from build123d import *

# Parameters (mm, degrees)
BOSS_EXTRUDE1_DEPTH      = 88.9
BOSS_EXTRUDE1_DEPTH_BACK = 88.9
SKETCH2_R                = 3.3782
CUT_EXTRUDE2_DEPTH       = 163.899847125
SKETCH5_R                = 14.2875
SKETCH5_R_2              = 3.3782
CUT_EXTRUDE3_DEPTH       = 164.564592404
BOSS_EXTRUDE3_START      = -19.05
BOSS_EXTRUDE3_DEPTH      = 201.6125
CONVERT_SOLID1_START     = -88.9
CONVERT_SOLID1_DEPTH     = 177.8
CONVERT_SOLID1_START_2   = -103.98125
CONVERT_SOLID1_2_DEPTH   = 201.6125
CONVERT_SOLID1_3_DEPTH   = 177.8
CONVERT_SOLID1_4_DEPTH   = 201.6125
SKETCH7_R                = 3.3782
CUT_EXTRUDE4_DEPTH       = 185.298076003


# Read off the part's stored shape, not the designer's step: Convert-Solid1
with BuildPart() as part:
    # Sketch1 → Boss-Extrude1 (new, two sides: drawn at the far end of the back side and taken through both)
    with BuildSketch(Plane(origin=(0, 0, 0), x_dir=(0, 0, -1), z_dir=(1, 0, 0)).offset(-BOSS_EXTRUDE1_DEPTH_BACK)):
        Polygon((-132.55625, -29.4132), (-132.55625, -32.5882), (-113.50625, -32.5882), (-113.50625, 0), (113.50625, 0), (113.50625, -32.5882), (132.55625, -32.5882), (132.55625, -29.4132), (116.68125, -29.4132), (116.68125, 3.175), (-116.68125, 3.175), (-116.68125, -29.4132), align=None)
    extrude(amount=BOSS_EXTRUDE1_DEPTH + BOSS_EXTRUDE1_DEPTH_BACK)

    # Sketch2 → Cut-Extrude2 (cut, through all)
    with BuildSketch(Plane(origin=(0, -29.4132, 0), x_dir=(1, 0, 0), z_dir=(0, 1, 0))):
        with Locations(Location((-76.2, -124.61875, 0), (0, 0, 270))):
            Circle(SKETCH2_R)
        with Locations(Location((0, -124.61875, 0), (0, 0, 270))):
            Circle(SKETCH2_R)
        with Locations(Location((76.2, -124.61875, 0), (0, 0, 270))):
            Circle(SKETCH2_R)
        with Locations(Location((76.2, 124.61875, 0), (0, 0, 90))):
            Circle(SKETCH2_R)
        with Locations(Location((0, 124.61875, 0), (0, 0, 90))):
            Circle(SKETCH2_R)
        with Locations(Location((-76.2, 124.61875, 0), (0, 0, 90))):
            Circle(SKETCH2_R)
    extrude(amount=-CUT_EXTRUDE2_DEPTH, mode=Mode.SUBTRACT)

    # Sketch5 → Cut-Extrude3 (cut, through all)
    with BuildSketch(Plane(origin=(0, 3.175, 0), x_dir=(1, 0, 0), z_dir=(0, 1, 0))):
        with Locations(Location((0, 12.7, 0), (0, 0, 270))):
            Circle(SKETCH5_R)
        with Locations(Location((-70.612, 83.312, 0), (0, 0, 270))):
            Circle(SKETCH5_R_2)
        with Locations(Location((70.612, 83.312, 0), (0, 0, 270))):
            Circle(SKETCH5_R_2)
        with Locations(Location((70.612, -57.912, 0), (0, 0, 270))):
            Circle(SKETCH5_R_2)
        with Locations(Location((-70.612, -57.912, 0), (0, 0, 270))):
            Circle(SKETCH5_R_2)
    extrude(amount=-CUT_EXTRUDE3_DEPTH, mode=Mode.SUBTRACT)

    # Sketch6 → Boss-Extrude3 (add)
    with BuildSketch(Plane.XY.offset(116.68125).offset(BOSS_EXTRUDE3_START)):
        Polygon((88.9, 3.175), (107.95, 3.175), (107.95, -29.4132), (123.825, -29.4132), (123.825, -32.5882), (104.775, -32.5882), (104.775, 0), (88.9, 0), align=None)
        Polygon((-88.9, 0), (-88.9, 3.175), (-107.95, 3.175), (-107.95, -29.4132), (-123.825, -29.4132), (-123.825, -32.5882), (-104.775, -32.5882), (-104.775, 0), align=None)
    extrude(amount=-BOSS_EXTRUDE3_DEPTH)

    # Convert-Solid1 outline → Convert-Solid1 (add)
    with BuildSketch(Plane.YZ.offset(CONVERT_SOLID1_START)):
        with BuildLine():
            Line((-29.4132, -116.68125), (-29.4132, -117.95125))
            ThreePointArc((-29.4132, -117.95125), (-29.041225612, -117.053224388), (-28.1432, -116.68125))
            Line((-28.1432, -116.68125), (-29.4132, -116.68125))
        make_face()
        with BuildLine():
            Line((0, -113.50625), (0, -112.23625))
            ThreePointArc((0, -112.23625), (-0.371974388, -113.134275612), (-1.27, -113.50625))
            Line((-1.27, -113.50625), (0, -113.50625))
        make_face()
        with BuildLine():
            ThreePointArc((-1.27, 113.50625), (-0.371974388, 113.134275612), (0, 112.23625))
            Line((0, 112.23625), (0, 113.50625))
            Line((0, 113.50625), (-1.27, 113.50625))
        make_face()
        with BuildLine():
            Line((-29.4132, 116.68125), (-28.1432, 116.68125))
            ThreePointArc((-28.1432, 116.68125), (-29.041225612, 117.053224388), (-29.4132, 117.95125))
            Line((-29.4132, 117.95125), (-29.4132, 116.68125))
        make_face()
    extrude(amount=CONVERT_SOLID1_DEPTH)

    # Convert-Solid1 2 outline → Convert-Solid1 2 (add)
    with BuildSketch(Plane.XY.offset(CONVERT_SOLID1_START_2)):
        with BuildLine():
            Line((107.95, -29.4132), (109.22, -29.4132))
            ThreePointArc((109.22, -29.4132), (108.321974388, -29.041225612), (107.95, -28.1432))
            Line((107.95, -28.1432), (107.95, -29.4132))
        make_face()
        with BuildLine():
            Line((-107.95, -29.4132), (-107.95, -28.1432))
            ThreePointArc((-107.95, -28.1432), (-108.321974388, -29.041225612), (-109.22, -29.4132))
            Line((-109.22, -29.4132), (-107.95, -29.4132))
        make_face()
        with BuildLine():
            ThreePointArc((-104.775, -1.27), (-104.403025612, -0.371974388), (-103.505, 0))
            Line((-103.505, 0), (-104.775, 0))
            Line((-104.775, 0), (-104.775, -1.27))
        make_face()
        with BuildLine():
            ThreePointArc((103.505, 0), (104.403025612, -0.371974388), (104.775, -1.27))
            Line((104.775, -1.27), (104.775, 0))
            Line((104.775, 0), (103.505, 0))
        make_face()
    extrude(amount=CONVERT_SOLID1_2_DEPTH)

    # Convert-Solid1 3 outline → Convert-Solid1 3 (cut)
    with BuildSketch(Plane.YZ.offset(CONVERT_SOLID1_START)):
        with BuildLine():
            ThreePointArc((-32.5882, -117.95125), (-31.286289642, -114.808160358), (-28.1432, -113.50625))
            Line((-28.1432, -113.50625), (-32.5882, -113.50625))
            Line((-32.5882, -113.50625), (-32.5882, -117.95125))
        make_face()
        with BuildLine():
            Line((-32.5882, 113.50625), (-28.1432, 113.50625))
            ThreePointArc((-28.1432, 113.50625), (-31.286289642, 114.808160358), (-32.5882, 117.95125))
            Line((-32.5882, 117.95125), (-32.5882, 113.50625))
        make_face()
        with BuildLine():
            ThreePointArc((-1.27, 116.68125), (1.873089642, 115.379339642), (3.175, 112.23625))
            Line((3.175, 112.23625), (3.175, 116.68125))
            Line((3.175, 116.68125), (-1.27, 116.68125))
        make_face()
        with BuildLine():
            ThreePointArc((3.175, -112.23625), (1.873089642, -115.379339642), (-1.27, -116.68125))
            Line((-1.27, -116.68125), (3.175, -116.68125))
            Line((3.175, -116.68125), (3.175, -112.23625))
        make_face()
    extrude(amount=CONVERT_SOLID1_3_DEPTH, mode=Mode.SUBTRACT)

    # Convert-Solid1 4 outline → Convert-Solid1 4 (cut)
    with BuildSketch(Plane.XY.offset(CONVERT_SOLID1_START_2)):
        with BuildLine():
            ThreePointArc((-107.95, -1.27), (-106.648089642, 1.873089642), (-103.505, 3.175))
            Line((-103.505, 3.175), (-107.95, 3.175))
            Line((-107.95, 3.175), (-107.95, -1.27))
        make_face()
        with BuildLine():
            ThreePointArc((103.505, 3.175), (106.648089642, 1.873089642), (107.95, -1.27))
            Line((107.95, -1.27), (107.95, 3.175))
            Line((107.95, 3.175), (103.505, 3.175))
        make_face()
        with BuildLine():
            Line((104.775, -32.5882), (109.22, -32.5882))
            ThreePointArc((109.22, -32.5882), (106.076910358, -31.286289642), (104.775, -28.1432))
            Line((104.775, -28.1432), (104.775, -32.5882))
        make_face()
        with BuildLine():
            Line((-104.775, -32.5882), (-104.775, -28.1432))
            ThreePointArc((-104.775, -28.1432), (-106.076910358, -31.286289642), (-109.22, -32.5882))
            Line((-109.22, -32.5882), (-104.775, -32.5882))
        make_face()
    extrude(amount=CONVERT_SOLID1_4_DEPTH, mode=Mode.SUBTRACT)

    # Sketch7 → Cut-Extrude4 (cut, through all)
    with BuildSketch(Plane(origin=(0, -29.4132, 0), x_dir=(1, 0, 0), z_dir=(0, 1, 0))):
        with Locations(Location((115.8875, -84.93125, 0), (0, 0, 270))):
            Circle(SKETCH7_R)
        with Locations(Location((115.8875, 3.175, 0), (0, 0, 270))):
            Circle(SKETCH7_R)
        with Locations(Location((115.8875, 91.28125, 0), (0, 0, 270))):
            Circle(SKETCH7_R)
        with Locations(Location((-115.8875, -84.93125, 0), (0, 0, 90))):
            Circle(SKETCH7_R)
        with Locations(Location((-115.8875, 3.175, 0), (0, 0, 90))):
            Circle(SKETCH7_R)
        with Locations(Location((-115.8875, 91.28125, 0), (0, 0, 90))):
            Circle(SKETCH7_R)
    extrude(amount=-CUT_EXTRUDE4_DEPTH, mode=Mode.SUBTRACT)


solid = part.part
Geometry: final body of the model. Coordinates: model frame, mm. A direction names the side the tool comes from. Coordinates: 2 decimals unless noted, no trailing zeros. Order: outer loops, then holes, each group sorted by start corner. A loop starts at its lowest first (then second) coordinate and runs counter-clockwise, first axis right, second up.
(1) Section query C-C (x = -22). Return the cut outline in (y, z) (3 decimals), plus the area to 3 significant figures.
(2) Section query A-A (y = -23.5). Return the cut outline in (x, z) (3 decimals), plus the area to 3 significant figures.
(3) Section query D-D (z = 93.5). Return the cut outline in (x, y) (3 decimals), plus the area to 3 significant figures.
(4) First-contact query: pin 1 (9 mm diameter, centred on x = 70.612, z = -83.312, fed in from -Y); pin 2 (1.5 mm diameter, centred on x = -29, y = -8.5, fed in from +Z); pin 3 (6 mm diameter, centred on y = -18, z = 31.5, fed in from -X). Flat tips, straight axial feed; report the tip coordinate or a pass-through.
(5) Material intervals for probe 1 along Z at (x, y) = (-57, -25.5); probe 2 along X at (y, z) = (-21, -14.5) (3 decimals); probe 3 along Z at (x, y) = (-76, -31), sorted ascending.
(6) Draft query along X for faces 1 (the face through (67.615, 1.61, 59.471)), 2 (the face through (-88.9, -16, -116)), 3 (the face through (-120, -32.588, -2)). Return one class per face: pulls with the +X half, pulls with the -X half, needs draft (parallel to the pull), parting line crosses it, or undercut.
(7) Access query for faces 4 (the face through (107.95, -15, -2)), 5 (the face through (-1.2, -29.413, 128.4)), 6 (the face through (-88.9, -15, 115)). Directions: +Z, -Z, +X, -X, +Y, -Y. A direction counts if a zero-diameter tool reaches every point of the face in a straight line with its end or side. Return the directions, or none.
Solution:
1. outline: (-32.588, -132.556) - (-29.413, -132.556) - (-29.413, -117.951) arc R1.27 cw to (-28.143, -116.681) - (-1.27, -116.681) arc R4.445 ccw to (3.175, -112.236) - (3.175, 112.236) arc R4.445 ccw to (-1.27, 116.681) - (-28.143, 116.681) arc R1.27 cw to (-29.413, 117.951) - (-29.413, 132.556) - (-32.588, 132.556) - (-32.588, 117.951) arc R4.445 ccw to (-28.143, 113.506) - (-1.27, 113.506) arc R1.27 cw to (0, 112.236) - (0, -112.236) arc R1.27 cw to (-1.27, -113.506) - (-28.143, -113.506) arc R4.445 ccw to (-32.588, -117.951) - close
1. area: 1,030 mm2
2. outline: (-107.95, -103.981) - (-104.775, -103.981) - (-104.775, 97.631) - (-107.95, 97.631) - close; (-88.9, -116.681) - (88.9, -116.681) - (88.9, -113.506) - (-88.9, -113.506) - close; (-88.9, 113.506) - (88.9, 113.506) - (88.9, 116.681) - (-88.9, 116.681) - close; (104.775, -103.981) - (107.95, -103.981) - (107.95, 97.631) - (104.775, 97.631) - close
2. area: 2,410 mm2
3. outline: (-123.825, -32.588) - (-109.22, -32.588) arc R4.445 ccw to (-104.775, -28.143) - (-104.775, -1.27) arc R1.27 cw to (-103.505, 0) - (103.505, 0) arc R1.27 cw to (104.775, -1.27) - (104.775, -28.143) arc R4.445 ccw to (109.22, -32.588) - (123.825, -32.588) - (123.825, -29.413) - (109.22, -29.413) arc R1.27 cw to (107.95, -28.143) - (107.95, -1.27) arc R4.445 ccw to (103.505, 3.175) - (-103.505, 3.175) arc R4.445 ccw to (-107.95, -1.27) - (-107.95, -28.143) arc R1.27 cw to (-109.22, -29.413) - (-123.825, -29.413) - close
3. area: 978 mm2
4. pin 1: stops at y = 0
4. pin 2: stops at z = 116.68
4. pin 3: stops at x = -107.95
5. probe 1: z = -116.68 to -113.51, 113.51 to 116.68
5. probe 2: x = -107.95 to -104.775, 104.775 to 107.95
5. probe 3: z = -132.56 to -127.99, -121.25 to -114.55, 114.55 to 121.25, 127.99 to 132.56
6. face 1: undercut
6. face 2: pulls with the -X half
6. face 3: needs draft
7. face 4: +Z, -Z, +X, +Y
7. face 5: +Z, +X, -X, +Y
7. face 6: +Z, -X, +Y, -Y
